Source: CAD feature listing. Evaluate the final solid. Frame: model axes, mm. A direction names the side the tool comes from. Coordinates: 2 decimals unless noted, no trailing zeros. Order: outer loops, then holes, each group sorted by start corner. A loop starts at its lowest first (then second) coordinate and runs counter-clockwise, first axis right, second up.
```python
from build123d import *

# Parameters (mm, degrees)
BOSS_EXTRUDE1_DEPTH      = 3
M3_CLEARANCE_HOLE1_D     = 3.2
M3_CLEARANCE_HOLE2_D     = 3.2
F_4_0_4_DIAMETER_HOLE1_D = 4
EXTRUDE_THIN1_DEPTH      = 3
BOSS_EXTRUDE4_START      = -3
BOSS_EXTRUDE4_DEPTH      = 3
FILLET4_R                = 3


with BuildPart() as part:
    # Sketch2 → Boss-Extrude1 (new body)
    with BuildSketch(Plane(origin=(0, 0, 0), x_dir=(1, 0, 0), z_dir=(0, 1, 0))):
        with BuildLine():
            Line((-6.15, 41.5), (14.85, 41.5))
            Line((14.85, 41.5), (14.85, 15.5))
            Line((14.85, 15.5), (13.66471398, -0.982645329))
            ThreePointArc((13.66471398, -0.982645329), (9.687362902, -9.687362902), (0.982645329, -13.66471398))
            Line((0.982645329, -13.66471398), (-15.5, -14.85))
            Line((-15.5, -14.85), (-41.5, -14.85))
            Line((-41.5, -14.85), (-41.5, 6.15))
            Line((-41.5, 6.15), (-6.15, 41.5))
        make_face()
    extrude(amount=BOSS_EXTRUDE1_DEPTH)

    # M3 Clearance Hole1 (through all)
    with Locations(Plane(origin=(0, 3, 0), x_dir=(1, 0, 0), z_dir=(0, 1, 0))):
        with Locations((-38.5, 3.15), (-18.5, 3.15), (-18.5, -11.85), (-38.5, -11.85), (-3.15, 18.5), (-3.15, 38.5), (11.85, 38.5), (11.85, 18.5)):
            Hole(M3_CLEARANCE_HOLE1_D / 2)

    # M3 Clearance Hole2 (through all)
    with Locations(Plane(origin=(0, 3, 0), x_dir=(1, 0, 0), z_dir=(0, 1, 0))):
        with Locations((-2.329371406, 8.693332437), (6.363961031, 6.363961031), (8.693332437, -2.329371406), (2.329371406, -8.693332437), (-6.363961031, -6.363961031), (-8.693332437, 2.329371406)):
            Hole(M3_CLEARANCE_HOLE2_D / 2)

    # Ø4.0 (4) Diameter Hole1 (through all)
    with Locations(Plane(origin=(0, 3, 0), x_dir=(1, 0, 0), z_dir=(0, 1, 0))):
        with Locations((0, 0)):
            Hole(F_4_0_4_DIAMETER_HOLE1_D / 2)



with BuildPart() as body_2:
    # Sketch11 → Extrude-Thin1 (new body)
    with BuildSketch(Plane(origin=(0, 3, 0), x_dir=(1, 0, 0), z_dir=(0, 1, 0))):
        with BuildLine():
            Line((-7, -24), (7, -24))
            ThreePointArc((7, -24), (11.242640687, -25.757359313), (13, -30))
            Line((13, -30), (13, -34))
            ThreePointArc((13, -34), (11.242640687, -38.242640687), (7, -40))
            Line((7, -40), (-7, -40))
            ThreePointArc((-7, -40), (-11.242640687, -38.242640687), (-13, -34))
            Line((-13, -34), (-13, -30))
            ThreePointArc((-13, -30), (-11.242640687, -25.757359313), (-7, -24))
        make_face()
        with BuildLine():
            Line((-7, -27), (7, -27))
            ThreePointArc((7, -27), (9.121320344, -27.878679656), (10, -30))
            Line((10, -30), (10, -34))
            ThreePointArc((10, -34), (9.121320344, -36.121320344), (7, -37))
            Line((7, -37), (-7, -37))
            ThreePointArc((-7, -37), (-9.121320344, -36.121320344), (-10, -34))
            Line((-10, -34), (-10, -30))
            ThreePointArc((-10, -30), (-9.121320344, -27.878679656), (-7, -27))
        make_face(mode=Mode.SUBTRACT)
    extrude(amount=-EXTRUDE_THIN1_DEPTH)


with BuildPart() as part_1:
    add(part.part)

    add(body_2.part)  # Boss-Extrude4 merges body 2
    # Sketch12 → Boss-Extrude4 (add)
    with BuildSketch(Plane(origin=(0, 3, 0), x_dir=(1, 0, 0), z_dir=(0, 1, 0)).offset(BOSS_EXTRUDE4_START)):
        with BuildLine():
            Line((11.242640687, -38.242640687), (24.742640687, -24.742640687))
            Line((24.742640687, -24.742640687), (9.687362902, -9.687362902))
            ThreePointArc((9.687362902, -9.687362902), (5.693601612, -12.460854733), (0.982645329, -13.66471398))
            Line((0.982645329, -13.66471398), (-15.5, -14.85))
            Line((-15.5, -14.85), (-23.260783473, -14.85))
            Line((-23.260783473, -14.85), (-12.368766817, -36.678869699))
            ThreePointArc((-12.368766817, -36.678869699), (-12.84005997, -35.376117563), (-13, -34))
            Line((-13, -34), (-13, -30))
            ThreePointArc((-13, -30), (-11.242640687, -25.757359313), (-7, -24))
            Line((-7, -24), (7, -24))
            ThreePointArc((7, -24), (11.242640687, -25.757359313), (13, -30))
            Line((13, -30), (13, -34))
            ThreePointArc((13, -34), (12.543277195, -36.296100594), (11.242640687, -38.242640687))
        make_face()
    extrude(amount=BOSS_EXTRUDE4_DEPTH)

    # Mirror4: part across plane


with BuildPart() as part_2:
    add(part_1.part)
    add(part_1.part.mirror(Plane(origin=(0, 0, 0), x_dir=(0.7071067811865478, 0, 0.7071067811865472), z_dir=(-0.7071067811865475, 0, 0.7071067811865477))))

    # Fillet4
    fillet4_edges = [part_2.edges().sort_by_distance(p)[0] for p in [
        (-23.260783473, 1.5, 14.85),
        (-6.15, 1.5, -41.5),
        (14.85, 1.5, -41.5),
        (-41.5, 1.5, 14.85),
        (-41.5, 1.5, -6.15),
        (14.85, 1.5, -23.260783473),
    ]]
    fillet(fillet4_edges, radius=FILLET4_R)


solid = part_2.part
```
1. Draft query along Z for faces 3 (the face through (-38.15, 1.48, 13.41)), 4 (the face through (-10.117, 1.521, 39.127)), 5 (the face through (-6.04, 1.52, -41.28)), 6 (the face through (14.85, 1, -32)). Return one class per face: released by +Z, released by -Z, zero draft, split by the parting line, or undercut.
Findings:
face 3: undercut
face 4: released by +Z
face 5: released by -Z
face 6: zero draft
2. Section query C-C on x = -18.5. Return loops of the section in (y, z), plus the area to 3 significant figures.
Findings:
outline: (0, -29.15) - (3, -29.15) - (3, -4.75) - (0, -4.75) - close; (0, -1.55) - (3, -1.55) - (3, 10.25) - (0, 10.25) - close; (0, 13.45) - (3, 13.45) - (3, 24.39) - (0, 24.39) - close
area: 141 mm2
3. Access query for faces 1 (the face through (27.86, 1.52, 9.1)), 2 (the face through (-1, 3, 8)). Directions: +Z, -Z, +X, -X, +Y, -Y. A direction counts if a zero-diameter tool reaches every point of the face in a straight line with its end or side. Return the directions, or none.
Findings:
face 1: +Y, -Y
face 2: +Z, -Z, +X, -X, +Y
4. Section query B-B on z = -18.5. Return loops of the section in (x, y).
Findings:
outline: (-29.15, 0) - (-4.75, 0) - (-4.75, 3) - (-29.15, 3) - close; (-1.55, 0) - (10.25, 0) - (10.25, 3) - (-1.55, 3) - close; (13.45, 0) - (24.39, 0) - (24.39, 3) - (13.45, 3) - close
5. Section query D-D on z = -29. Return loops of the section in (x, y), plus the area to 4 significant figures.
Findings:
outline: (-18.65, 0) - (14.85, 0) - (14.85, 3) - (-18.65, 3) - close
area: 100.5 mm2
6. Section query A-A on x = 31. Return loops of the section in (y, z), plus the area to 3 significant figures.
Findings:
outline: (0, -15.2) - (3, -15.2) - (3, -10) - (0, -10) - close; (0, 10) - (3, 10) - (3, 18.49) - (0, 18.49) - close
area: 41.1 mm2
7. Pin query (flat end, axial travel): P1, Ø8, axis at x = 2, z = 8, coming from the +Y side; P2, Ø1, axis at x = -31.5, y = 0.5, coming from the -Z side; P3, Ø3, axis at x = -3.15, z = -18.5, coming from the +Y side; P4, Ø0.9, axis at x = -29.5, y = 2, coming from the +Z side. Return the tip coordinate at first contact, or that it passes through.
Findings:
P1: stops at y = 3
P2: stops at z = -16.65
P3: passes through
P4: stops at z = 14.85
8. Ray query, line 1 (X direction, y = 0.3, z = 7); line 2 (Z direction, x = -3.15, y = 2.3); line 3 (X direction, y = 0.45, z = 3.5). Return the intervals inside material, ascending.
Findings:
line 1: x = -41.5 to -7.83, -4.9 to 27, 37 to 40
line 2: z = -41.5 to -40.1, -36.9 to -20.1, -16.9 to -10.07, -7.32 to 27, 37 to 40
line 3: x = -41.5 to 7.6, 9.78 to 27, 37 to 40
